The drawing under review shows one solid part. Ordinate dimensions are in mm from its lowest x, y, z. Give positions to 0.01 mm unless a question says otherwise; leave off trailing zeros. Loops run counter-clockwise (first coordinate to the right, second up) from the corner with the lowest first, then second, coordinate; pieces in that order, holes last. Notation, with made-up numbers: (7.5, 13) - (19.5, 13) arc R36 ccw to (19.5, 52) - close; hole circle Ø5 at (-32, 83). An arc over 180 degrees is marked (long way). Return JSON: item names as keys, results as strings. Group by question number.
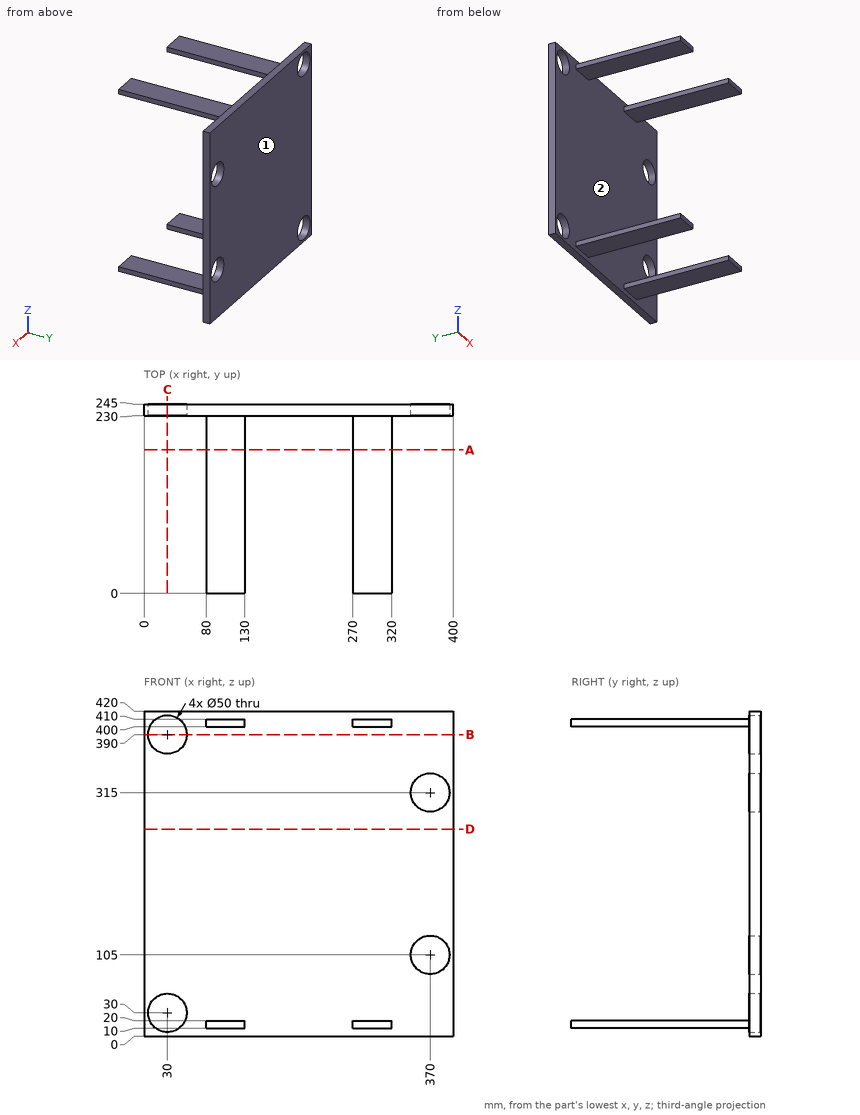
1) We need section C-C, the plane x = 30. Write out the cut boundary in (y, z), plus the area to 3 significant figures.
2) We need section B-B, the plane z = 390. Write out the cut boundary in (x, y), plus the area to 3 significant figures.
3) For pin 1 Ø5 at (y, z) = (88.5, 15.5) entering from +X; pin 2 Ø25 at (x, y) = (105.5, 94.5) entering from +Z; pin 3 Ø12 at (x, y) = (304, 105.5) entering from -Z, all flat-tipped, find the tip position at first contact; note any pin that passes through.
4) Draft analysis for pull direction Z (two halves, no side actions). For the marked faces 1 and 2, state which applies: +Z half, -Z half, draft (parallel to the pull), parting line (faces both ways), or undercut.
5) We need section A-A, the plane y = 185.5. Write out the cut boundary in (x, z), plus the area to 3 significant figures.
6) To check wall thickness, follow line 1 (Z direction, x = 30, y = 240); line 2 (X direction, y = 239, z = 315); line 3 (Y direction, x = 33.5, z = 326). State the ranges of each line that lie inside material, in increasing order.
7) We need section D-D, the plane z = 267.5. Write out the cut boundary in (x, y).
Findings:
{
 "1": {"outline": "(230, 0) - (245, 0) - (245, 5) - (230, 5) - close; (230, 55) - (245, 55) - (245, 365) - (230, 365) - close; (230, 415) - (245, 415) - (245, 420) - (230, 420) - close", "area": "4,800 mm^2"},
 "2": {"outline": "(0, 230) - (5, 230) - (5, 245) - (0, 245) - close; (55, 230) - (400, 230) - (400, 245) - (55, 245) - close", "area": "5,250 mm^2"},
 "3": {"pin 1": "stops at x = 320", "pin 2": "stops at z = 410", "pin 3": "stops at z = 10"},
 "4": {"face 1": "draft", "face 2": "undercut"},
 "5": {"outline": "(80, 10) - (130, 10) - (130, 20) - (80, 20) - close; (80, 400) - (130, 400) - (130, 410) - (80, 410) - close; (270, 10) - (320, 10) - (320, 20) - (270, 20) - close; (270, 400) - (320, 400) - (320, 410) - (270, 410) - close", "area": "2,000 mm^2"},
 "6": {"line 1": "z = 0 to 5, 55 to 365, 415 to 420", "line 2": "x = 0 to 345, 395 to 400", "line 3": "y = 230 to 245"},
 "7": {"outline": "(0, 230) - (400, 230) - (400, 245) - (0, 245) - close"}
}
